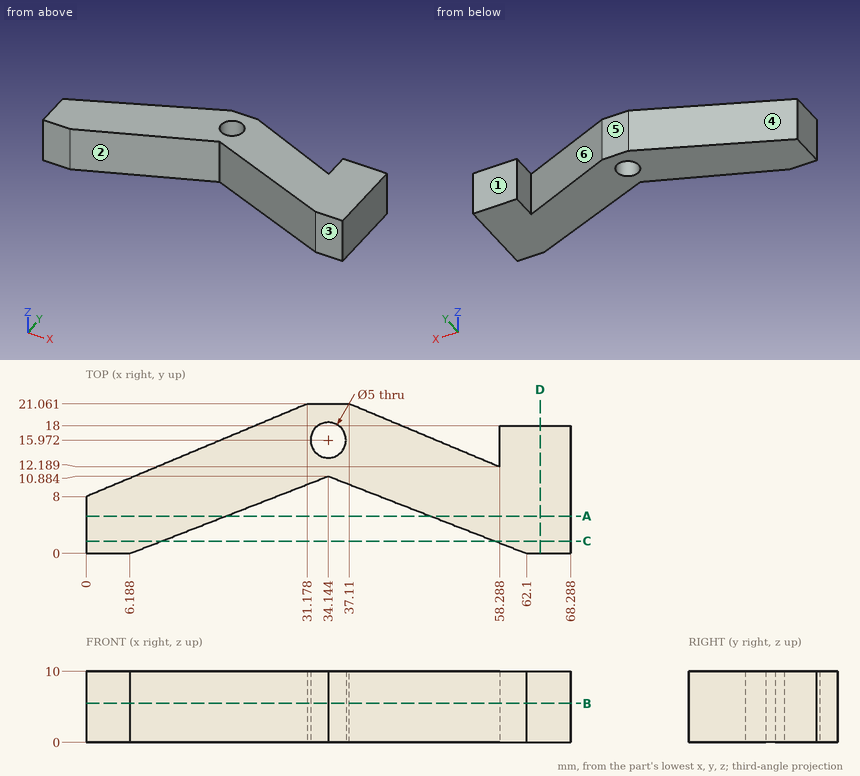
Geometry check sheet. Reference: drawing and pictorial views, mm from the part's lowest x, y, z. A direction names the side the tool comes from. Round coordinates to 2 decimals unless told otherwise and drop trailing zeros. Loops run counter-clockwise (first coordinate to the right, second up) from the corner with the lowest first, then second, coordinate; pieces in that order, holes last. Notation, with made-up numbers: (15.5, 1) - (40.5, 1) arc R26 cw to (40.5, 24) - close; hole circle Ø1 at (-21.5, -35). An arc over 180 degrees is marked (long way). Answer in a Markdown table with one row per item. Add a question column.
Q1. Section check C-C on y = 1.75. Enter the section's corners in (x, z) (1 decimal), plus the area to 3 significant figures.
Q2. Section check A-A on y = 5.25. Enter the section's corners in (x, z) (1 decimal).
Q3. Material ranges on line 1 (Y direction, x = 65.5, z = 5); line 2 (X direction, y = 19, z = 6.75) (1 decimal); line 3 (Y direction, x = 27, z = 5.5), recorded low to high.
Q4. Gauge pin test, flat ends, axial feed: pin 1 (1.7 mm diameter, centred on y = 15.5, z = 7.5, fed in from -X) (1 decimal); pin 2 (4 mm diameter, centred on x = 52.5, z = 6, fed in from +Y); pin 3 (1.5 mm diameter, centred on x = 46, z = 7.5, fed in from -Y). Record the tip position at first contact, or that the pin passes through.
Q5. Tool access check on the marked faces 1, 2 and 3. Record the directions out of +Z, -Z, +X, -X, +Y, -Y that give a thin tool (end or side, any length) a straight path to the whole face; none if there is none.
Q6. Section check D-D on x = 64. Enter the section's corners in (y, z).
Q7. Release check for a two-part mould opening along X. For the marked faces 4, 5 and 6 record: pulls with the +X half, pulls with the -X half, needs draft (parallel to the pull), parting line crosses it, or undercut.
Q8. Section check B-B on z = 5.5. Enter the section's corners in (x, y).
Found:
| question | item | result |
|---|---|---|
| 1 | outline | (0, 0) - (10.7, 0) - (10.7, 10) - (0, 10) - close; (57.6, 0) - (68.3, 0) - (68.3, 10) - (57.6, 10) - close |
| 1 | area | 214 mm² |
| 2 | outline | (0, 0) - (19.7, 0) - (19.7, 10) - (0, 10) - close; (48.6, 0) - (68.3, 0) - (68.3, 10) - (48.6, 10) - close |
| 3 | line 1 | y = 0 to 18 |
| 3 | line 2 | x = 26.3 to 42 |
| 3 | line 3 | y = 8.1 to 19.31 |
| 4 | pin 1 | stops at x = 15.9 |
| 4 | pin 2 | stops at y = 15.45 |
| 4 | pin 3 | stops at y = 5.98 |
| 5 | face 1 | +Z, -Z, +X, +Y |
| 5 | face 2 | +Z, -Z, -Y |
| 5 | face 3 | +Z, -Z, +X, -X, -Y |
| 6 | outline | (0, 0) - (18, 0) - (18, 10) - (0, 10) - close |
| 7 | face 4 | pulls with the -X half |
| 7 | face 5 | needs draft |
| 7 | face 6 | undercut |
| 8 | outline | (0, 0) - (6.19, 0) - (34.14, 10.88) - (62.1, 0) - (68.29, 0) - (68.29, 18) - (58.29, 18) - (58.29, 12.19) - (37.11, 21.06) - (31.18, 21.06) - (0, 8) - close; hole circle Ø5 at (34.14, 15.97) |
